Work out the finished part from the listing and answer in its coordinate system (mm). Face numbers are marked on the shaded views. A direction names the side the tool comes from. Coordinates: 2 decimals unless noted, no trailing zeros. Order: outer loops, then holes, each group sorted by start corner. A loop starts at its lowest first (then second) coordinate and runs counter-clockwise, first axis right, second up. Notation, with made-up numbers: M -6.5,24.25 L 47.5,24.25 A12 ccw 47.5,39.25 Z; hole C 85,82.5 d10. An arc over 180 degrees is marked long. Answer in a Markdown table with one row per item. Add a question column.
Item 1: The part is cut by section C-C (y = -2.5). Write down the section's boundary in (x, z).
Item 2: Flat-ended cylindrical pins translate along their axes: pin 1 Ø3.5 at (x, z) = (184, 45) entering from -Y; pin 2 Ø1.5 at (y, z) = (25, 40.5) entering from -X; pin 3 Ø4 at (x, y) = (158, 6.5) entering from -Z; pin 4 Ø1 at (x, y) = (137, 15.5) entering from -Z. Find the tip coordinate at first contact, or state that the pin passes through.
Item 3: The part is cut by section A-A (x = 94). Write down the section's boundary in (y, z), then the cut area to 3 significant figures.
Item 4: The part is cut by section B-B (z = 11.5). Write down the section's boundary in (x, y).
Item 5: The part is cut by section D-D (x = 172). Write down the section's boundary in (y, z).
Item 6: Which of the six approach directions +Z, -Z, +X, -X, +Y, -Y give full straight-line access (tool end or side, diameter ignored) to the marked faces 1 and 2?
Item 7: Consider line 1 (Z direction, x = 184, y = 24.5); line 2 (X direction, y = 25.1, z = 45); line 3 (X direction, y = 25, z = -45). Determine where each line is inside the solid, lowest interval first. Write a range as from..to.
from build123d import *

# Parameters (mm, degrees)
BOSS_EXTRUDE1_DEPTH = 3
FILLET3_R           = 5
FILLET2_R           = 1
SKETCH2_R           = 1.5
CUT_EXTRUDE1_DEPTH  = 3
SKETCH5_R           = 10
BOSS_EXTRUDE2_DEPTH = 40
SKETCH3_R           = 6
CUT_EXTRUDE3_DEPTH  = 3
CUT_EXTRUDE3_TAPER  = -5
SKETCH6_R           = 2
BOSS_EXTRUDE3_DEPTH = 8
BOSS_EXTRUDE3_TAPER = 1
SKETCH7_R           = 1
BOSS_EXTRUDE4_DEPTH = 0.5


with BuildPart() as part:
    # Sketch1 → Boss-Extrude1 (new body)
    with BuildSketch(Plane(origin=(0, 23, 0), x_dir=(1, 0, 0), z_dir=(0, 1, 0))):
        Polygon((98.305417602, 50), (98.305417602, 28.219474586), (89, 28.219474586), (89, -35.308001182), (91.659783805, -35.308001182), (91.659783805, -50), (97.650210801, -50), (189, -50), (189, 50), align=None)
    extrude(amount=BOSS_EXTRUDE1_DEPTH)

    # Fillet3
    fillet3_edges = [part.edges().sort_by_distance(p)[0] for p in [
        (189, 24.5, 50),
        (91.659783805, 24.5, 50),
        (98.305417602, 24.5, -50),
        (189, 24.5, -50),
    ]]
    fillet(fillet3_edges, radius=FILLET3_R)

    # Fillet2
    fillet2_edges = [part.edges().sort_by_distance(p)[0] for p in [
        (91.659783805, 24.5, 35.308001182),
        (89, 24.5, 35.308001182),
        (89, 24.5, -28.219474586),
        (98.305417602, 24.5, -28.219474586),
    ]]
    fillet(fillet2_edges, radius=FILLET2_R)

    # Sketch2 → Cut-Extrude1 (cut)
    with BuildSketch(Plane(origin=(0, 23, 0), x_dir=(1, 0, 0), z_dir=(0, 1, 0))):
        with Locations((184, -45)):
            Circle(SKETCH2_R)
        with Locations((94, -30.308001182)):
            Circle(SKETCH2_R)
        with Locations((94, 23.219474586)):
            Circle(SKETCH2_R)
        with Locations((184, 45)):
            Circle(SKETCH2_R)
    extrude(amount=CUT_EXTRUDE1_DEPTH, mode=Mode.SUBTRACT)

    # Sketch5 → Boss-Extrude2 (add)
    with BuildSketch(Plane(origin=(0, 23, 0), x_dir=(1, 0, 0), z_dir=(0, 1, 0))):
        with Locations((149, 0)):
            Circle(SKETCH5_R)
    extrude(amount=-BOSS_EXTRUDE2_DEPTH)

    # Sketch3 → Cut-Extrude3 (cut)
    with BuildSketch(Plane(origin=(0, 23, 0), x_dir=(1, 0, 0), z_dir=(0, 1, 0))):
        with Locations((149, 0)):
            Circle(SKETCH3_R)
    extrude(amount=CUT_EXTRUDE3_DEPTH, taper=CUT_EXTRUDE3_TAPER, mode=Mode.SUBTRACT)

    # Sketch6 → Boss-Extrude3 (add)
    with BuildSketch(Plane(origin=(0, 23, 0), x_dir=(1, 0, 0), z_dir=(0, 1, 0))):
        with Locations((149, 0)):
            Circle(SKETCH6_R)
    extrude(amount=BOSS_EXTRUDE3_DEPTH, taper=BOSS_EXTRUDE3_TAPER)

    # Sketch7 → Boss-Extrude4 (add)
    with BuildSketch(Plane(origin=(0, 26, 0), x_dir=(1, 0, 0), z_dir=(0, 1, 0))):
        with Locations((115.065320099, 35)):
            Circle(SKETCH7_R)
    extrude(amount=BOSS_EXTRUDE4_DEPTH)


solid = part.part
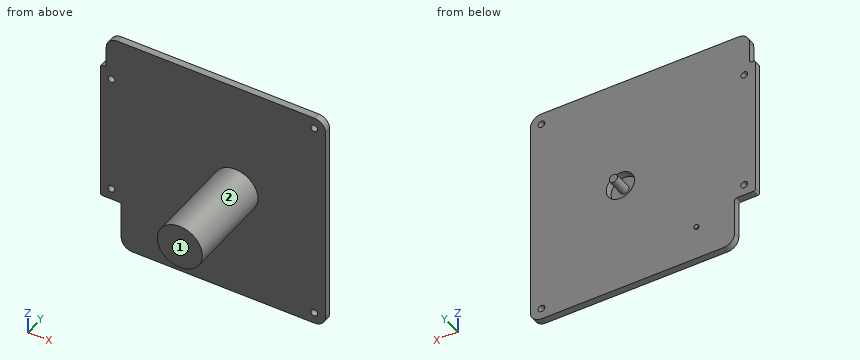
Reply:
| question | item | result |
|---|---|---|
| 1 | outline | C 149,0 d20 |
| 2 | pin 1 | stops at y = 23 |
| 2 | pin 2 | stops at x = 91.66 |
| 2 | pin 3 | stops at z = -7.14 |
| 2 | pin 4 | passes through |
| 3 | outline | M 23,-28.22 L 26,-28.22 L 26,-24.72 L 23,-24.72 Z; M 23,-21.72 L 26,-21.72 L 26,28.81 L 23,28.81 Z; M 23,31.81 L 26,31.81 L 26,49.23 L 23,49.23 Z |
| 3 | area | 214 mm2 |
| 4 | outline | M 89,23 L 189,23 L 189,26 L 89,26 Z |
| 5 | outline | M 23,-50 L 26,-50 L 26,50 L 23,50 Z |
| 6 | face 1 | +Z, -Z, +X, -X, -Y |
| 6 | face 2 | -Y |
| 7 | line 1 | z = -50..-46.5, -43.5..43.5, 46.5..50 |
| 7 | line 2 | x = 91.66..182.5, 185.5..189 |
| 7 | line 3 | x = 98.31..182.5, 185.5..189 |
